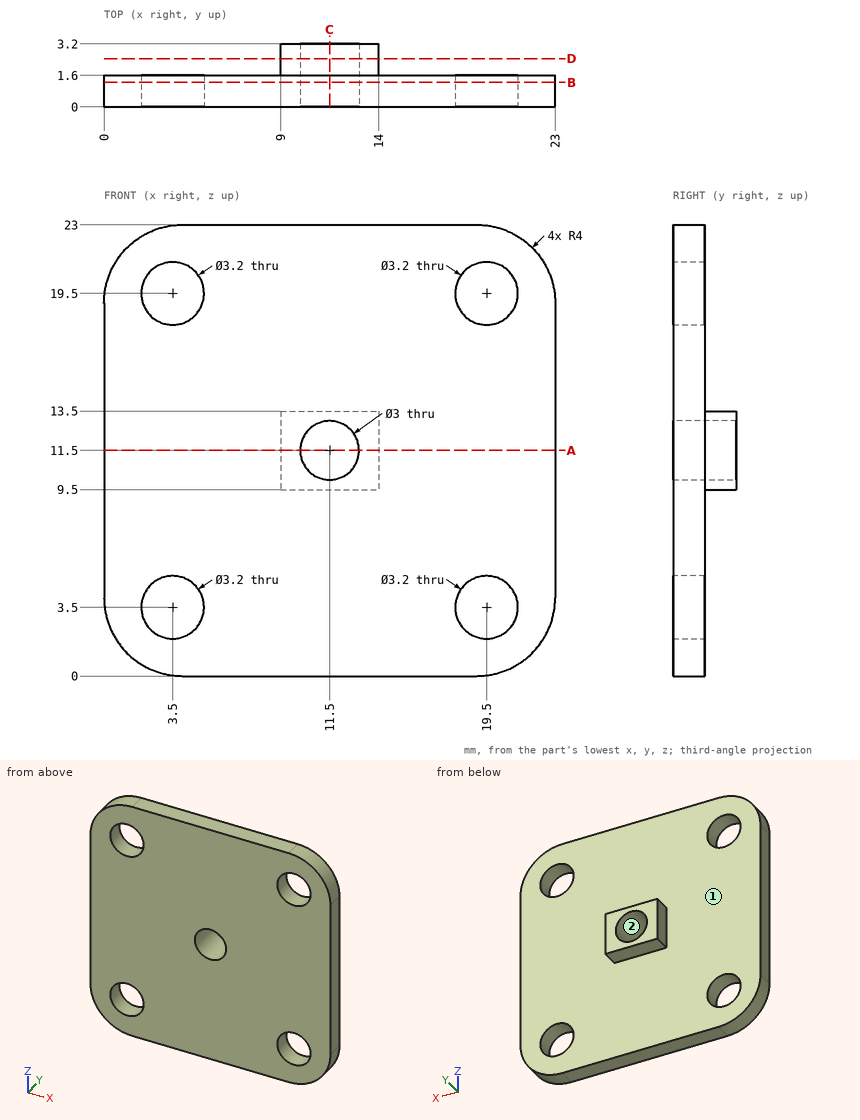
Source: three-view drawing plus pictorial views. Frame: mm from the lowest corner of the part. Coordinates: 2 decimals unless noted, no trailing zeros. Loops run counter-clockwise (first coordinate to the right, second up) from the corner with the lowest first, then second, coordinate; pieces in that order, holes last. Notation, with made-up numbers: M -2.75,-36.5 L 54.25,-36.5 A22 cw 54.25,-12.5 Z; hole C 83,35 d10. An arc over 180 degrees is marked long. Use CSV: the item, a comma, the result in double quotes.
(1) Cut plane B-B on y = 1.25. Return loops of the section in (x, z), and give its area (3 significant figures).
Answers follow:
outline,"M 0,4 A4 ccw 4,0 L 19,0 A4 ccw 23,4 L 23,19 A4 ccw 19,23 L 4,23 A4 ccw 0,19 Z; hole C 3.5,3.5 d3.2; hole C 3.5,19.5 d3.2; hole C 11.5,11.5 d3; hole C 19.5,3.5 d3.2; hole C 19.5,19.5 d3.2"
area,"476 mm²"
(2) Contact query for flat-ended pins moving along their axis: pin 1 (1.5 mm diameter, centred on x = 12.5, z = 16, fed in from -Y); pin 2 (4 mm diameter, centred on x = 3.5, z = 19.5, fed in from +Y); pin 3 (1.3 mm diameter, centred on x = 11.5, y = 2.5, fed in from -Z); pin 4 (0.8 mm diameter, centred on x = 12, y = 2.5, fed in from +Z). Output: stop coordinate, or through.
Answers follow:
pin 1,"y = 0"
pin 2,"y = 1.6"
pin 3,"z = 9.5"
pin 4,"z = 13.5"
(3) Cut plane A-A on z = 11.5. Return loops of the section in (x, y), and give its area (3 significant figures).
Answers follow:
outline,"M 0,0 L 10,0 L 10,3.2 L 9,3.2 L 9,1.6 L 0,1.6 Z; M 13,0 L 23,0 L 23,1.6 L 14,1.6 L 14,3.2 L 13,3.2 Z"
area,"35.2 mm²"
(4) Draft query along Z for the marked faces 1 and 2. Return one class per face: pulls with the +Z half, pulls with the -Z half, needs draft (parallel to the pull), parting line crosses it, or undercut.
Answers follow:
face 1,"needs draft"
face 2,"undercut"
(5) Cut plane D-D on y = 2.45. Return loops of the section in (x, z).
Answers follow:
outline,"M 9,9.5 L 14,9.5 L 14,13.5 L 9,13.5 Z; hole C 11.5,11.5 d3"
(6) Cut plane C-C on x = 11.5. Return loops of the section in (y, z), and give its area (3 significant figures).
Answers follow:
outline,"M 0,0 L 1.6,0 L 1.6,9.5 L 3.2,9.5 L 3.2,10 L 0,10 Z; M 0,13 L 3.2,13 L 3.2,13.5 L 1.6,13.5 L 1.6,23 L 0,23 Z"
area,"33.6 mm²"
(7) Line query: line 1 (X direction, y = 0.6, z = 3.5); line 2 (X direction, y = 0.95, z = 4); line 3 (X direction, y = 1.25, z = 11.5). Output: solid intervals per line, ascending. Write a range as [from, to].
Answers follow:
line 1,"[0.03, 1.9], [5.1, 17.9], [21.1, 22.97]"
line 2,"[0, 1.98], [5.02, 17.98], [21.02, 23]"
line 3,"[0, 10], [13, 23]"
